Part model, mm, in its own coordinate system. Give positions to 0.01 mm unless a question says otherwise; leave off trailing zeros. Loops run counter-clockwise (first coordinate to the right, second up) from the corner with the lowest first, then second, coordinate; pieces in that order, holes last. Notation, with made-up numbers: (-38, 83.5) -> (-21, 83.5) arc R31 ccw to (-21, 109.5) -> close; hole circle Ø3 at (72, -13). An arc over 180 degrees is marked (long way). Write item = value, one per line.
from build123d import *

# Parameters (mm, degrees)
SKETCH1_R        = 60
SKETCH1_R_2      = 43.5
EXTRUSION1_DEPTH = 60
EXTRUSION3_START = -60
EXTRUSION3_DEPTH = 60


with BuildPart() as part:
    # Sketch1 → Extrusion1 (new body)
    with BuildSketch(Plane.XY):
        Circle(SKETCH1_R)
        Circle(SKETCH1_R_2, mode=Mode.SUBTRACT)
    extrude(amount=EXTRUSION1_DEPTH)

    # Sketch3 → Extrusion3 (cut)
    with BuildSketch(Plane.XY.offset(60).offset(EXTRUSION3_START)):
        with BuildLine():
            Line((-0.5, 48.5), (-0.5, 43.497126342))
            ThreePointArc((-0.5, 43.497126342), (0, 43.5), (0.5, 43.497126342))
            Line((0.5, 43.497126342), (0.5, 48.5))
            Line((0.5, 48.5), (-0.5, 48.5))
        make_face()
    extrude(amount=EXTRUSION3_DEPTH, mode=Mode.SUBTRACT)


solid = part.part
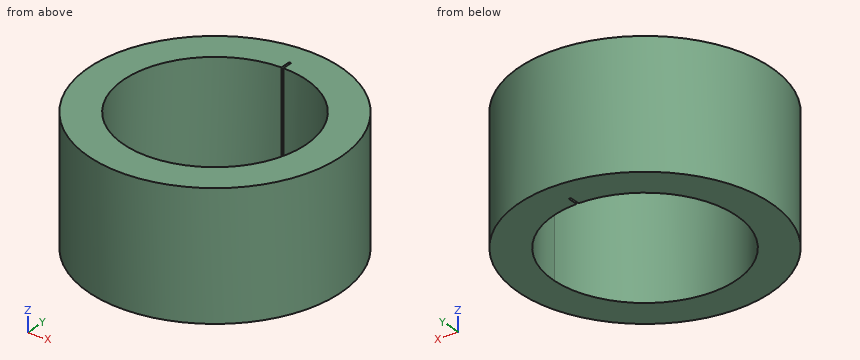
1) Drill centre lines: line 1 along Y through (x, z) = (0, 37); line 2 along X through (y, z) = (-7.5, 39.5); line 3 along Y through (x, z) = (27.5, 40.5). Where is each one in solid material? Low to high. Write a range as [from, to].
Resolved:
line_1 = [-60, -43.5], [48.5, 60]
line_2 = [-59.53, -42.85], [42.85, 59.53]
line_3 = [-53.33, -33.7], [33.7, 53.33]
2) Slice it at A-A, the plane y = 12.5. List the corners of the cut face in (x, z).
Resolved:
outline = (-58.68, 0) -> (-41.67, 0) -> (-41.67, 60) -> (-58.68, 60) -> close; (41.67, 0) -> (58.68, 0) -> (58.68, 60) -> (41.67, 60) -> close
3) Slice it at C-C, the plane z = 22.5. List the corners of the cut face in (x, y).
Resolved:
outline = circle Ø120 at (0, 0); hole (-0.5, 43.5) arc R43.5 ccw (long way) to (0.5, 43.5) -> (0.5, 48.5) -> (-0.5, 48.5) -> close
4) Slice it at B-B, the plane x = 37. List the corners of the cut face in (y, z).
Resolved:
outline = (-47.23, 0) -> (-22.87, 0) -> (-22.87, 60) -> (-47.23, 60) -> close; (22.87, 0) -> (47.23, 0) -> (47.23, 60) -> (22.87, 60) -> close
5) Drop flat-ended pins along their axis: P1, Ø2.5, axis at y = 46.5, z = 43.5, coming from the -X side; P2, Ø1, axis at x = 14, z = 49.5, coming from the -Y side; P3, Ø5, axis at y = 10.5, z = 24, coming from the +X side. Give the stop position or say it passes through.
Resolved:
P1 = -39.4
P2 = -58.46
P3 = 59.46
6) Slice it at D-D, the plane x = -48.5. List the corners of the cut face in (y, z), and give its area (3 significant figures).
Resolved:
outline = (-35.32, 0) -> (35.32, 0) -> (35.32, 60) -> (-35.32, 60) -> close
area = 4,240 mm²
